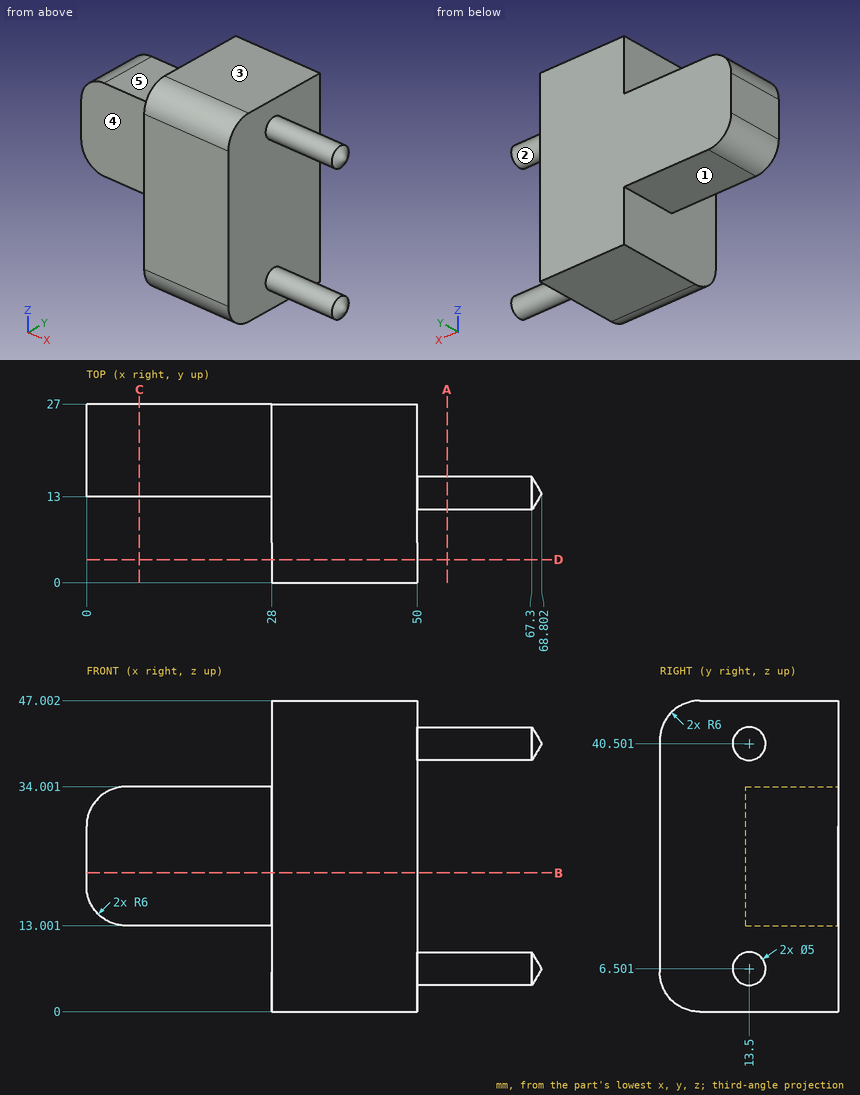
Source: three-view drawing plus pictorial views. Frame: mm from the lowest corner of the part. A direction names the side the tool comes from. Give positions to 0.01 mm unless a question says otherwise; leave off trailing zeros. Order: outer loops, then holes, each group sorted by start corner. A loop starts at its lowest first (then second) coordinate and runs counter-clockwise, first axis right, second up. Notation, with made-up numbers: (36, -4.75) -> (51, -4.75) arc R25 cw to (51, 8.25) -> close; hole circle Ø6 at (-9, 37). An arc over 180 degrees is marked (long way). Put each result on its own line as item: value.
Q1. Section D-D, the plane y = 3.5. Return loops of the section in (x, z).
Here are the results:
outline: (28, 0.55) -> (50, 0.55) -> (50, 46.46) -> (28, 46.46) -> close
Q2. Section A-A, the plane x = 54.5. Return loops of the section in (y, z).
Here are the results:
outline: circle Ø5 at (13.5, 6.5); circle Ø5 at (13.5, 40.5)
Q3. Section C-C, the plane x = 8. Return loops of the section in (y, z), then the cut area to 3 significant figures.
Here are the results:
outline: (13, 13) -> (27, 13) -> (27, 34) -> (13, 34) -> close
area: 294 mm^2
Q4. Section B-B, the plane z = 21. Return loops of the section in (x, y).
Here are the results:
outline: (0, 13) -> (28, 13) -> (28, 0) -> (50, 0) -> (50, 27) -> (0, 27) -> close
Q5. Material intervals for L1, parallel to X at y = 25, z = 3; L2, parallel to Y at x = 26.5, z = 13.5; L3, parallel to X at y = 20.25, z = 20, sorted ascending.
Here are the results:
L1: x = 28 to 50
L2: y = 13 to 27
L3: x = 0 to 50
Q6. Pin query (flat end, axial travel): pin 1 (11 mm diameter, centred on x = 14, y = 21, fed in from -Z); pin 2 (6.5 mm diameter, centred on x = 11.5, z = 27, fed in from -Y); pin 3 (10 mm diameter, centred on y = 10, z = 34.5, fed in from +X); pin 4 (5 mm diameter, centred on x = 20.5, y = 10, fed in from -Z). Return the tip coordinate at first contact, or that it passes through.
Here are the results:
pin 1: stops at z = 13
pin 2: stops at y = 13
pin 3: stops at x = 67.63
pin 4: passes through
Q7. Reachability of the marked faces 1, 2, 3, 4 and 5 from +Z, -Z, +X, -X, +Y, -Y: full face, straight path, thin tool, end or side. Return the list, or none.
Here are the results:
face 1: -Z, -X, +Y, -Y
face 2: +X
face 3: +Z, +X, -X, +Y, -Y
face 4: +Z, -Z, -X, -Y
face 5: +Z, -X, +Y, -Y
